```python
from build123d import *

# Parameters (mm, degrees)
F4_R     = 4.7625
F5_DEPTH = 9.525
F7_R     = 1.5875
F8_DEPTH = 22.225


# Not quite as in the source:
# - a fillet or chamfer that OpenCascade refuses, or shapes differently, is made with other operations: its cross-section is extruded or revolved along the edge and cut away or added


with BuildPart() as f2:
    # F0 (on Front) → F2 (revolve)
    with BuildSketch(Plane.XZ):
        Polygon((0, 50.8), (0, 0), (24.5263007426, 20.1624173125), (24.5263007426, 23.8990907568), (8.2719810307, 23.8990907568), (8.2719810307, 50.8), align=None)
    revolve(axis=Axis((0, 0, 25.4), (0, 0, -1)))

    # F3: fillet of radius 5.08 on 1 edges, made by hand

    # F3_s1 → F3_t2 (revolve, cut)
    with BuildSketch(Plane.XZ):
        with BuildLine():
            ThreePointArc((24.5263007426, 20.1624173125), (22.7079011169, 22.8583047213), (19.6271300205, 23.8990907568))
            Line((19.6271300205, 23.8990907568), (24.5263007426, 23.8990907568))
            Line((24.5263007426, 23.8990907568), (24.5263007426, 20.1624173125))
        make_face()
    revolve(axis=Axis((0, 0, 23.8990907568), (0, 0, -1)), mode=Mode.SUBTRACT)

    # F4 (on face) → F5 (cut)
    with BuildSketch(Plane.XY.offset(50.8)):
        Circle(F4_R)
    extrude(amount=-F5_DEPTH, mode=Mode.SUBTRACT)

    # F6: chamfer of 5.08 on 1 edges, made by hand

    # F6_s1 → F6_t2 (revolve, cut)
    with BuildSketch(Plane.XZ):
        Polygon((8.2719810307, 45.72), (3.1919810307, 50.8), (8.2719810307, 50.8), align=None)
    revolve(axis=Axis((0, 0, 50.8), (0, 0, -1)), mode=Mode.SUBTRACT)

    # F7 (on Top) → F8 (cut)
    with BuildSketch(Plane.XY):
        Circle(F7_R)
    extrude(amount=F8_DEPTH, mode=Mode.SUBTRACT)


solid = f2.part
```
Here's how the part is built. I have some questions about the finished solid (model axes, mm). A direction names the side the tool comes from. Round coordinates to 2 decimals unless told otherwise and drop trailing zeros. Loops run counter-clockwise (first coordinate to the right, second up) from the corner with the lowest first, then second, coordinate; pieces in that order, holes last.
1. If I drill on probe 1 along Y at (x, z) = (0, 45); probe 2 along X at (y, z) = (0, 10); probe 3 along X at (y, z) = (3.5, 44.5), over which ranges is the centre line in solid material (lowest first)?
Answers:
probe 1: y = -8.27 to -4.76, 4.76 to 8.27
probe 2: x = -12.16 to -1.59, 1.59 to 12.16
probe 3: x = -7.5 to -3.23, 3.23 to 7.5
2. For faces 5 (the face through (0, 0, 41.275)), 6 (the face through (5.314, -1.673, 4.58)), which set-ups out of +Z, -Z, +X, -X, +Y, -Y let a thin tool reach every point of the face, with its end or its side?
Answers:
face 5: +Z
face 6: -Z
3. Suppose I cut it at A-A, the plane y = 0. Please give me the cut outline in (x, z) (1 decimal), and give its area (3 significant figures).
Answers:
outline: (-24.5, 20.2) - (-1.6, 1.3) - (-1.6, 22.2) - (1.6, 22.2) - (1.6, 1.3) - (24.5, 20.2) arc R5.1 ccw to (19.6, 23.9) - (8.3, 23.9) - (8.3, 45.7) - (4.8, 49.2) - (4.8, 41.3) - (-4.8, 41.3) - (-4.8, 49.2) - (-8.3, 45.7) - (-8.3, 23.9) - (-19.6, 23.9) arc R5.1 ccw to start
area: 931 mm2
4. Suppose I cut it at D-D, the plane z = 6.5. Please give me the cut outline in (x, y) (1 decimal).
Answers:
outline: circle Ø15.8 at (0, 0); hole circle Ø3.2 at (0, 0)
5. Thinking about a two-plate mould opening in X: for faces 1 (the face through (0, 0, 22.225)), 2 (the face through (-6.564, 5.033, 34.962)), 3 (the face through (-0.34, -1.55, 11.62)), 4 (the face through (-0.27, 8.45, 23.899)), which applies, released by +X, released by -X, zero draft, split by the parting line, or undercut?
Answers:
face 1: undercut
face 2: split by the parting line
face 3: undercut
face 4: zero draft
6. Suppose I cut it at C-C, the plane z = 37. Please give me the cut outline in (x, y), and give its area (3 significant figures).
Answers:
outline: circle Ø16.54 at (0, 0)
area: 215 mm2
7. Will these pins go through, and if not, where does the flat tip stop? pin 1 (3.5 mm diameter, centred on x = 0, y = 0.5, fed in from -Z); pin 2 (5 mm diameter, centred on x = -1, y = -1, fed in from +Z) (3 decimals); pin 3 (2 mm diameter, centred on y = -14, z = 18.5, fed in from +X); pin 4 (6 mm diameter, centred on x = 0, z = 7, fed in from +Y).
Answers:
pin 1: stops at z = 1.31
pin 2: stops at z = 41.275
pin 3: stops at x = 19.31
pin 4: stops at y = 12.16
